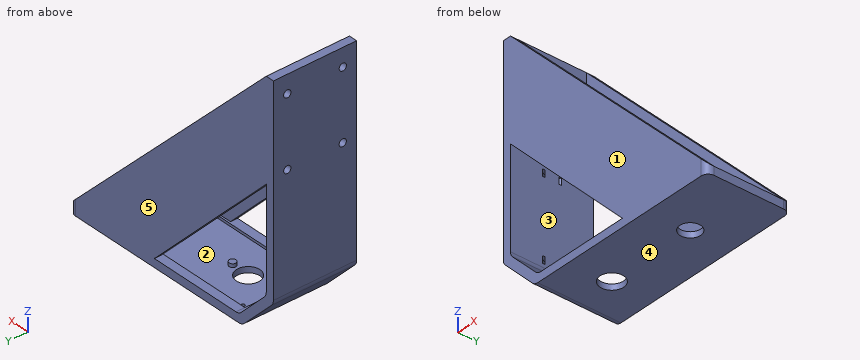
```python
from build123d import *

# Parameters (mm, degrees)
F1_DEPTH     = 60
F2_W         = 137
F2_H         = 47.15
F3_DEPTH     = 1.85
F5_D         = 2.5
F5_DEPTH     = 3
F5_TIP       = 0.7510757738
F4_R         = 2.425
F6_DEPTH     = 2.5
F8_D         = 5.25
F9_T1_DEPTH  = 60
F9_T6_DEPTH  = 60
F9_T12_DEPTH = 60
F9_T18_DEPTH = 60
F9_T25_DEPTH = 60
F9_T31_DEPTH = 60
F9_T34_DEPTH = 72.0912564168
F9_T36_DEPTH = 72.7642259517
F4_R_2       = 8.5
F4_R_3       = 7.5
F10_DEPTH    = 25
F12_DEPTH    = 5.1
F14_DEPTH    = 5.1
F15_R        = 5
F18_DEPTH    = 2.5
F21_DEPTH    = 2.5


# Not quite as in the source:
# - a fillet or chamfer that OpenCascade refuses, or shapes differently, is made with other operations: its cross-section is extruded or revolved along the edge and cut away or added
# - a feature names something its author has since deleted; it is built from what else it names


with BuildPart() as f1:
    # F0 (on Front) → F1 (new body)
    with BuildSketch(Plane.XZ):
        Polygon((-22.8349631621, 174.7265526258), (-28.8349631621, 174.7265526258), (-28.8349631621, 29.7265526258), (-28.8349631621, 27.3083013424), (-2.5528451903, 0), (0, 0), (141.95, 0), (141.95, 6), (0, 6), (-22.8349631621, 29.7265526258), (-22.8349631621, 151.506786451), align=None)
    extrude(amount=F1_DEPTH)

    # F2 (on face) → F3 (cut)
    with BuildSketch(Plane.XY.offset(6)):
        with Locations((70.975, -30)):
            Rectangle(F2_W, F2_H)
    extrude(amount=-F3_DEPTH, mode=Mode.SUBTRACT)

    # F5
    with Locations(Plane.XY.offset(4.15)):
        with Locations((7.025, -8.9), (136.825, -8.9), (136.825, -51.1), (7.025, -51.1)):
            Hole(F5_D / 2, depth=F5_DEPTH)
            with Locations((0, 0, -(F5_DEPTH + F5_TIP / 2))):  # 118° drill point
                Cone(0, F5_D / 2, F5_TIP, mode=Mode.SUBTRACT)

    # F4 (on face) → F6 (join)
    with BuildSketch(Plane.XY.offset(4.15)):
        with Locations((40.225, -30)):
            Circle(F4_R)
        with Locations((120.925, -30)):
            Circle(F4_R)
    extrude(amount=F6_DEPTH)

    # F8 (through all)
    with Locations(Plane.YZ.offset(-22.8349631621)):
        with Locations((-50, 161.7265526258), (-10, 161.7265526258), (-10, 111.7265526258), (-50, 111.7265526258)):
            Hole(F8_D / 2)

    # F9: fillet of radius 6 on 4 edges, made by hand

    # F9_s2 → F9_t1 (join)
    with BuildSketch(Plane.XZ):
        with BuildLine():
            ThreePointArc((-22.8349631621, 32.1448039092), (-22.3999669258, 29.9018743269), (-21.1580521252, 27.9841667203))
            Line((-21.1580521252, 27.9841667203), (-22.8349631621, 29.7265526258))
            Line((-22.8349631621, 29.7265526258), (-22.8349631621, 32.1448039092))
        make_face()
    extrude(amount=F9_T1_DEPTH)


with BuildPart() as f9_tool4:
    # F9_s5 → F9_t6 (new body)
    with BuildSketch(Plane.XZ):
        with BuildLine():
            ThreePointArc((-1.7702437727, 7.8393628111), (0.2037840091, 6.4789573841), (2.5528451903, 6))
            Line((2.5528451903, 6), (0, 6))
            Line((0, 6), (-1.7702437727, 7.8393628111))
        make_face()
    extrude(amount=F9_T6_DEPTH)

    split(bisect_by=Plane.YZ.offset(2.475), keep=Keep.BOTTOM)

    split(bisect_by=Plane.XZ.offset(6.425), keep=Keep.BOTTOM)


with BuildPart() as f1_1:
    add(f1.part)

    # F9_t3: union F9_tool4
    add(f9_tool4.part)


with BuildPart() as f9_tool10:
    # F9_s11 → F9_t12 (new body)
    with BuildSketch(Plane.XZ):
        with BuildLine():
            ThreePointArc((-1.7702437727, 7.8393628111), (0.2037840091, 6.4789573841), (2.5528451903, 6))
            Line((2.5528451903, 6), (0, 6))
            Line((0, 6), (-1.7702437727, 7.8393628111))
        make_face()
    extrude(amount=F9_T12_DEPTH)

    split(bisect_by=Plane.YZ.offset(2.475), keep=Keep.TOP)

    split(bisect_by=Plane.XZ.offset(6.425), keep=Keep.BOTTOM)


with BuildPart() as f1_2:
    add(f1_1.part)

    # F9_t9: union F9_tool10
    add(f9_tool10.part)


with BuildPart() as f9_tool16:
    # F9_s17 → F9_t18 (new body)
    with BuildSketch(Plane.XZ):
        with BuildLine():
            ThreePointArc((-1.7702437727, 7.8393628111), (0.2037840091, 6.4789573841), (2.5528451903, 6))
            Line((2.5528451903, 6), (0, 6))
            Line((0, 6), (-1.7702437727, 7.8393628111))
        make_face()
    extrude(amount=F9_T18_DEPTH)

    split(bisect_by=Plane.XZ.offset(53.575), keep=Keep.BOTTOM)

    split(bisect_by=Plane.YZ.offset(2.475), keep=Keep.BOTTOM)

    split(bisect_by=Plane.XZ.offset(6.425), keep=Keep.TOP)


with BuildPart() as f1_3:
    add(f1_2.part)

    # F9_t15: union F9_tool16
    add(f9_tool16.part)


with BuildPart() as f9_tool23:
    # F9_s24 → F9_t25 (new body)
    with BuildSketch(Plane.XZ):
        with BuildLine():
            ThreePointArc((-1.7702437727, 7.8393628111), (0.2037840091, 6.4789573841), (2.5528451903, 6))
            Line((2.5528451903, 6), (0, 6))
            Line((0, 6), (-1.7702437727, 7.8393628111))
        make_face()
    extrude(amount=F9_T25_DEPTH)

    split(bisect_by=Plane.XZ.offset(53.575), keep=Keep.TOP)

    split(bisect_by=Plane.YZ.offset(2.475), keep=Keep.BOTTOM)


with BuildPart() as f1_4:
    add(f1_3.part)

    # F9_t22: union F9_tool23
    add(f9_tool23.part)


with BuildPart() as f9_tool29:
    # F9_s30 → F9_t31 (new body)
    with BuildSketch(Plane.XZ):
        with BuildLine():
            ThreePointArc((-1.7702437727, 7.8393628111), (0.2037840091, 6.4789573841), (2.5528451903, 6))
            Line((2.5528451903, 6), (0, 6))
            Line((0, 6), (-1.7702437727, 7.8393628111))
        make_face()
    extrude(amount=F9_T31_DEPTH)

    split(bisect_by=Plane.XZ.offset(53.575), keep=Keep.TOP)

    split(bisect_by=Plane.YZ.offset(2.475), keep=Keep.TOP)


with BuildPart() as f1_5:
    add(f1_4.part)

    # F9_t28: union F9_tool29
    add(f9_tool29.part)

    # F9_s35 → F9_t34 (cut)
    with BuildSketch(Plane.XZ.offset(-6.0456282084)):
        with BuildLine():
            ThreePointArc((-27.1580521252, 25.5659154369), (-28.3999669258, 27.4836230436), (-28.8349631621, 29.7265526258))
            Line((-28.8349631621, 29.7265526258), (-28.8349631621, 27.3083013424))
            Line((-28.8349631621, 27.3083013424), (-27.1580521252, 25.5659154369))
        make_face()
    extrude(amount=F9_T34_DEPTH, mode=Mode.SUBTRACT)

    # F9_s37 → F9_t36 (cut)
    with BuildSketch(Plane.XZ.offset(-6.3821129759)):
        with BuildLine():
            ThreePointArc((0, 0), (-2.3490611813, 0.4789573841), (-4.3230889631, 1.8393628111))
            Line((-4.3230889631, 1.8393628111), (-2.5528451903, 0))
            Line((-2.5528451903, 0), (0, 0))
        make_face()
    extrude(amount=F9_T36_DEPTH, mode=Mode.SUBTRACT)

    # F4 (on face) → F10 (cut)
    with BuildSketch(Plane.XY.offset(4.15)):
        with Locations((27.225, -30)):
            Circle(F4_R_2)
        with Locations((92.925, -30)):
            Circle(F4_R_3)
    extrude(amount=-F10_DEPTH, mode=Mode.SUBTRACT)

    # F11 (on face) → F12 (join)
    with BuildSketch(Plane(origin=(0, 0, 0), x_dir=(-1, 0, 0), z_dir=(0, 1, 0))):
        Polygon((22.8349631621, 103.4356782675), (22.8349631621, 174.7265526258), (-141.95, 6), (-70.9393056499, 6), align=None)
    extrude(amount=-F12_DEPTH)

    # F13 (on face) → F14 (join)
    with BuildSketch(Plane.XZ.offset(60)):
        Polygon((141.95, 6), (-22.8349631621, 174.7265526258), (-22.8349631621, 103.4356782675), (70.9393056499, 6), align=None)
    extrude(amount=-F14_DEPTH)

    # F15
    f15_edges = [f1_5.edges().sort_by_distance(p)[0] for p in [
        (141.95, -60, 3),
        (141.95, 0, 3),
    ]]
    fillet(f15_edges, radius=F15_R)

    # F17 (on line) → F18 (cut, symmetric)
    with BuildSketch(Plane.XY.offset(94.7265526258)):
        with BuildLine():
            Line((-21.5895338884, -23.119), (-22.8349631621, -23.119))
            ThreePointArc((-22.8349631621, -23.119), (-26.8349631621, -29.9997827216), (-22.8349631621, -36.8805654433))
            Line((-22.8349631621, -36.8805654433), (-21.7005347336, -36.8805654433))
            Line((-21.7005347336, -36.8805654433), (-21.7005347336, -34.9997827216))
            Line((-21.7005347336, -34.9997827216), (-22.8349631621, -34.9997827216))
            ThreePointArc((-22.8349631621, -34.9997827216), (-25.2691290512, -29.9997827216), (-22.8349631621, -24.9997827216))
            Line((-22.8349631621, -24.9997827216), (-21.5895338884, -24.9997827216))
            Line((-21.5895338884, -24.9997827216), (-21.5895338884, -23.119))
        make_face()
    extrude(amount=F18_DEPTH, both=True, mode=Mode.SUBTRACT)

    # F20 (on offset) → F21 (cut, symmetric)
    with BuildSketch(Plane.XY.offset(37.3265526258)):
        with BuildLine():
            Line((-21.657592603, -23.1192172784), (-22.9030218767, -23.1192172784))
            ThreePointArc((-22.9030218767, -23.1192172784), (-26.9030218767, -30), (-22.9030218767, -36.8807827216))
            Line((-22.9030218767, -36.8807827216), (-21.7685934482, -36.8807827216))
            Line((-21.7685934482, -36.8807827216), (-21.7685934482, -35))
            Line((-21.7685934482, -35), (-22.9030218767, -35))
            ThreePointArc((-22.9030218767, -35), (-25.3371877657, -30), (-22.9030218767, -25))
            Line((-22.9030218767, -25), (-21.657592603, -25))
            Line((-21.657592603, -25), (-21.657592603, -23.1192172784))
        make_face()
    extrude(amount=F21_DEPTH, both=True, mode=Mode.SUBTRACT)


solid = f1_5.part
```
Part model, mm, in its own coordinate system. Face numbers are marked on the shaded views. A direction names the side the tool comes from. Give positions to 0.01 mm unless a question says otherwise; leave off trailing zeros. Write each loop counter-clockwise with the first axis right and the second up, starting at its lowest first coordinate (ties: lowest second). Pieces come first, ordered by that corner, then holes. Notation, with made-up numbers: (69.5, -22.75) -> (77.5, -22.75) arc R15 ccw to (77.5, -9.75) -> close; hole circle Ø11 at (9.5, -34). An arc over 180 degrees is marked (long way). Put each result on its own line as item: value. Start each with the question number.
Item 1: Pin check, flat tips, straight feed: pin 1 Ø12 at (x, y) = (7.5, -17.5) entering from +Z; pin 2 Ø10 at (x, y) = (102, -41.5) entering from -Z; pin 3 Ø1.5 at (x, y) = (41, -31) entering from +Z; pin 4 Ø0.9 at (y, z) = (-28.5, 5.5) entering from -X. Stop position of each tip, or through.
Item 2: Cut at A-A (z = 19.5). List the corners of the cut face in (x, y).
Item 3: Wall check: L1, parallel to X at y = -51.1, z = 1.85 (3 decimals); L2, parallel to Y at x = 103.5, z = 41; L3, parallel to X at y = -51.1, z = 2.55 (3 decimals). Give the ranges that are in metal, low to high. Write a range as [from, to].
Item 4: Cut at D-D (z = 136). List the corners of the cut face in (x, y).
Item 5: Which spindle directions (+Z, -Z, +X, -X, +Y, -Y) get a long thin tool onto all of the face, cutting with end or side? Do the marked faces 1 and 2. Say none if no direction does.
Item 6: Cut at C-C (y = -30). State how many separate pieces and enclosed holes the cut face has, then the cut area to 3 significant figures.
Item 7: Cut at B-B (x = 54). List the corners of the cut face in (y, z) (3 decimals).
Item 8: Pull direction Y, two halves, no side cores. Call the marked faces 3, 4 and 5: pulls with the +Y half, pulls with the -Y half, needs draft (parallel to the pull), parting line crosses it, or undercut.
Answer list:
1. pin 1: stops at z = 6.09
1. pin 2: stops at z = 0
1. pin 3: stops at z = 6.65
1. pin 4: stops at x = -8.28
2. outline: (-21.32, -60) -> (-12.99, -60) -> (-12.99, 0) -> (-21.32, 0) -> close; (57.95, -60) -> (128.77, -60) -> (128.77, -54.9) -> (57.95, -54.9) -> close; (57.95, -5.1) -> (128.77, -5.1) -> (128.77, 0) -> (57.95, 0) -> close
3. L1: x = [-4.333, 5.775], [8.275, 135.575], [138.075, 141.95]
3. L2: y = [-60, -54.9], [-5.1, 0]
3. L3: x = [-5.007, 5.775], [8.275, 135.575], [138.075, 141.95]
4. outline: (-28.83, -60) -> (14.99, -60) -> (14.99, -54.9) -> (-22.83, -54.9) -> (-22.83, -5.1) -> (14.99, -5.1) -> (14.99, 0) -> (-28.83, 0) -> close
5. face 1: +Z, -Z, +X, -X, -Y
5. face 2: +Z
6. separate pieces: 3
6. enclosed holes: 2
6. area: 1,570 mm2
7. outline: (-60, 0) -> (0, 0) -> (0, 6) -> (-6.425, 6) -> (-6.425, 4.15) -> (-53.575, 4.15) -> (-53.575, 6) -> (-60, 6) -> close; (-60, 23.601) -> (-54.9, 23.601) -> (-54.9, 96.054) -> (-60, 96.054) -> close; (-5.1, 23.601) -> (0, 23.601) -> (0, 96.054) -> (-5.1, 96.054) -> close
8. face 3: undercut
8. face 4: needs draft
8. face 5: pulls with the +Y half
